Could you check a few things on this model? Use its own coordinates, in mm. A direction names the side the tool comes from. Round coordinates to 2 decimals unless told otherwise and drop trailing zeros. Write each loop counter-clockwise with the first axis right and the second up, starting at its lowest first coordinate (ties: lowest second). Pieces come first, ordered by that corner, then holes. Notation, with made-up numbers: M -33,52 L 15,52 A31 cw 15,84 Z; hole C 29,-6 d6. An arc over 180 degrees is marked long. One line per item, written item: value. Start each with the question number.
(1) I want a section at D-D on y = 31. Please give me the cut outline in (x, z), and give its area (3 significant figures).
(2) Thinking about a two-plate mould opening in Z: for faces 3 (the face through (1, 20, 0)), 4 (the face through (21.769, 25.677, 5.916)), 5 (the face through (1, 27, 63)), which applies, released by +Z, released by -Z, zero draft, split by the parting line, or undercut?
(3) I want a section at A-A on x = 19. Please give me the cut outline in (y, z), and give its area (3 significant figures).
(4) I want a section at B-B on y = 23.5. Please give me the cut outline in (x, z), and give its area (3 significant figures).
(5) I want a section at C-C on z = 67. Please give me the cut outline in (x, y), and give its area (3 significant figures).
(6) I'm going to push a flat-ended pin straight in: pin 1 Ø1.5 at (y, z) = (37.5, 10) entering from -X. Where does the tip first touch, or does it pass through?
(7) Which directions (+Z, -Z, +X, -X, +Y, -Y) give clear straight access to the entire face, cutting with the end or side of a thin tool? Please do faces 1 (the face through (-72, 6, 38)), 2 (the face through (1, 27, 12)).
(8) If I drill on L1, parallel to Y at x = -19, z = 4; L2, parallel to Z at x = 10.5, y = 14; L3, parallel to Y at x = -59.5, z = 40.5, over which ranges is the centre line in solid material (lowest first)?
```python
from build123d import *

# Parameters (mm, degrees)
SKETCH1_R                = 6
BOSS_EXTRUDE2_DEPTH      = 12
SKETCH3_W                = 144
SKETCH3_H                = 12
BOSS_EXTRUDE3_DEPTH      = 25.5
BOSS_EXTRUDE3_DEPTH_BACK = 25.5


with BuildPart() as part:
    # Sketch1 → Boss-Extrude2 (new body)
    with BuildSketch(Plane.XY):
        with BuildLine():
            Line((-32.5, 50), (32.5, 50))
            ThreePointArc((32.5, 50), (46.579087682, 25.10523588), (72, 12))
            Line((72, 12), (72, 0))
            Line((72, 0), (-72, 0))
            Line((-72, 0), (-72, 12))
            ThreePointArc((-72, 12), (-46.579087682, 25.10523588), (-32.5, 50))
        make_face()
        with Locations((19, 31)):
            Circle(SKETCH1_R, mode=Mode.SUBTRACT)
        with Locations((-19, 31)):
            Circle(SKETCH1_R, mode=Mode.SUBTRACT)
    extrude(amount=BOSS_EXTRUDE2_DEPTH)


with BuildPart() as body_2:
    # Mirror1: mirrored copy
    add(part.part.mirror(Plane.XY.offset(37.5)))


with BuildPart() as part_1:
    add(part.part)

    add(body_2.part)  # Boss-Extrude3 merges body 2
    # Sketch3 → Boss-Extrude3 (add, two sides)
    with BuildSketch(Plane.XY.offset(37.5)) as boss_extrude3_sk:
        with Locations((0, 6)):
            Rectangle(SKETCH3_W, SKETCH3_H)
    extrude(amount=BOSS_EXTRUDE3_DEPTH)
    extrude(boss_extrude3_sk.sketch, amount=-BOSS_EXTRUDE3_DEPTH_BACK)


solid = part_1.part
```
Found:
1. outline: M -41.35,0 L -25,0 L -25,12 L -41.35,12 Z; M -41.35,63 L -25,63 L -25,75 L -41.35,75 Z; M -13,0 L 13,0 L 13,12 L -13,12 Z; M -13,63 L 13,63 L 13,75 L -13,75 Z; M 25,0 L 41.35,0 L 41.35,12 L 25,12 Z; M 25,63 L 41.35,63 L 41.35,75 L 25,75 Z
1. area: 1,410 mm²
2. face 3: released by -Z
2. face 4: zero draft
2. face 5: undercut
3. outline: M 0,0 L 25,0 L 25,12 L 12,12 L 12,63 L 25,63 L 25,75 L 0,75 Z; M 37,0 L 50,0 L 50,12 L 37,12 Z; M 37,63 L 50,63 L 50,75 L 37,75 Z
3. area: 1,520 mm²
4. outline: M -48.33,0 L 48.33,0 L 48.33,12 L -48.33,12 Z; M -48.33,63 L 48.33,63 L 48.33,75 L -48.33,75 Z
4. area: 2,320 mm²
5. outline: M -72,0 L 72,0 L 72,12 A50 cw 32.5,50 L -32.5,50 A50 cw -72,12 Z; hole C -19,31 d12; hole C 19,31 d12
5. area: 4,860 mm²
6. pin 1: stops at x = -37.59
7. face 1: +Z, -Z, -X, +Y, -Y
7. face 2: +X, -X, +Y
8. L1: y = 0 to 25, 37 to 50
8. L2: z = 0 to 12, 63 to 75
8. L3: y = 0 to 12
